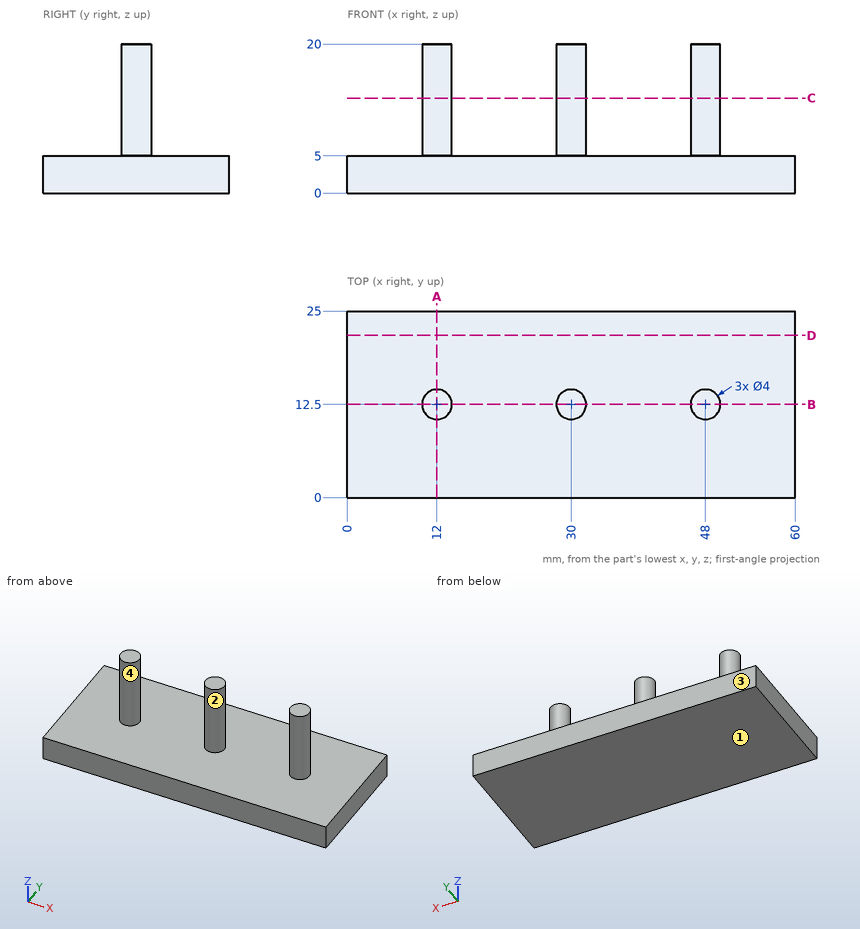
Could you check a few things on this drawing? It's one solid part, dimensions in mm from its lowest x, y, z. A direction names the side the tool comes from. Coordinates: 2 decimals unless noted, no trailing zeros. Loops run counter-clockwise (first coordinate to the right, second up) from the corner with the lowest first, then second, coordinate; pieces in that order, holes last. Notation, with made-up numbers: (-26.5, -11) - (-19.5, -11) arc R32 cw to (-19.5, 20) - close; hole circle Ø10 at (-33.75, -35.75). An arc over 180 degrees is marked (long way). Return JSON: item names as keys, results as strings. Group by question number.
Item 1: On a 3-axis mill with a long thin cutter (end or side, diameter ignored), from which of +Z, -Z, +X, -X, +Y, -Y can I reach the whole of each face in a straight line? I mean the marked faces 3 and 4. Say none if no direction works.
Item 2: If we section it at A-A on x = 12: Write out the boundary of the cut face in (y, z).
Item 3: If we section it at D-D on y = 21.75: Write out the boundary of the cut face in (x, z).
Item 4: If we section it at B-B on y = 12.5: Write out the boundary of the cut face in (x, z), and give its area (3 significant figures).
Item 5: I need wall thicknesses on line 1 (X direction, y = 13.5, z = 19); line 2 (X direction, y = 12.25, z = 10); line 3 (Z direction, x = 22.5, y = 13.25). Which ranges of each line are inside material? Lowest first, please. Write a range as from..to.
Item 6: Will these pins go through, and if not, where does the flat tip stop? P1, Ø12, axis at x = 21, z = 3.5, coming from the -Y side; P2, Ø4, axis at y = 11, z = 8, coming from the +X side; P3, Ø3, axis at x = 29.5, z = 17, coming from the -Y side; P4, Ø1.5, axis at x = 45, y = 16, coming from the +Z side.
Item 7: We'd pull the mould along X, two halves only. Please class the marked faces 1 and 2: +X half, -X half, draft (parallel to the pull), parting line (faces both ways), or undercut.
Item 8: If we section it at C-C on z = 12.75: Write out the boundary of the cut face in (x, y), and give its area (3 significant figures).
Calculated:
{
 "1": {"face 3": "+Z, -Z, +X, -X, +Y", "face 4": "+Z"},
 "2": {"outline": "(0, 0) - (25, 0) - (25, 5) - (14.5, 5) - (14.5, 20) - (10.5, 20) - (10.5, 5) - (0, 5) - close"},
 "3": {"outline": "(0, 0) - (60, 0) - (60, 5) - (0, 5) - close"},
 "4": {"outline": "(0, 0) - (60, 0) - (60, 5) - (50, 5) - (50, 20) - (46, 20) - (46, 5) - (32, 5) - (32, 20) - (28, 20) - (28, 5) - (14, 5) - (14, 20) - (10, 20) - (10, 5) - (0, 5) - close", "area": "480 mm^2"},
 "5": {"line 1": "x = 10.27..13.73, 28.27..31.73, 46.27..49.73", "line 2": "x = 10.02..13.98, 28.02..31.98, 46.02..49.98", "line 3": "z = 0..5"},
 "6": {"P1": "stops at y = 0", "P2": "stops at x = 50", "P3": "stops at y = 10.5", "P4": "stops at z = 5"},
 "7": {"face 1": "draft", "face 2": "undercut"},
 "8": {"outline": "circle Ø4 at (12, 12.5); circle Ø4 at (30, 12.5); circle Ø4 at (48, 12.5)", "area": "37.7 mm^2"}
}
